Verification items for this drawing (mm, ordinates from the low corner). Give positions to 0.01 mm unless a question says otherwise; leave off trailing zeros. Order: outer loops, then holes, each group sorted by start corner. A loop starts at its lowest first (then second) coordinate and runs counter-clockwise, first axis right, second up.
(1) Scan lines: L1, parallel to Z at x = 252, y = 0.35; L2, parallel to X at y = 0.55, z = 34.5. Record each from-to range of solid material in increasing order.
(2) Sectioned sample at A-A on y = 1.2. Record the cut outline in (x, z).
(3) Gauge pin test, flat ends, axial feed: pin 1 (1 mm diameter, centred on x = 91, z = 36.5, fed in from -Y); pin 2 (1.5 mm diameter, centred on y = 2, z = 88.5, fed in from +X); pin 3 (1.5 mm diameter, centred on y = 2, z = 88.5, fed in from -X). Record the tip position at first contact, or that the pin passes through.
(4) Sectioned sample at B-B on x = 169.5. Record the cut outline in (y, z), plus the area to 3 significant figures.
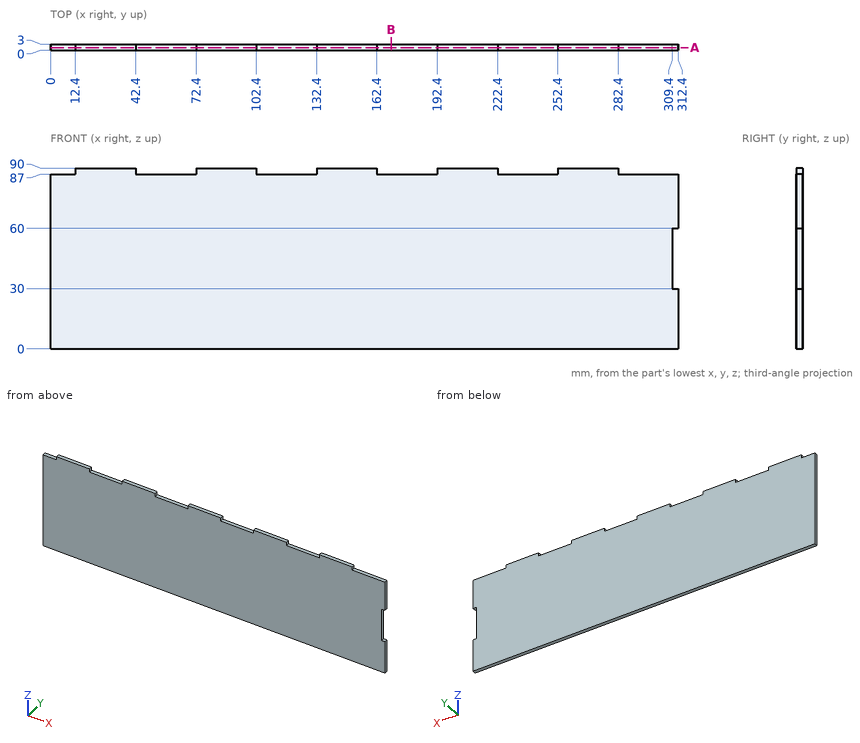
Ans:
1. L1: z = 0 to 87
1. L2: x = 0 to 309.4
2. outline: (0, 0) - (312.4, 0) - (312.4, 30) - (309.4, 30) - (309.4, 60) - (312.4, 60) - (312.4, 87) - (282.4, 87) - (282.4, 90) - (252.4, 90) - (252.4, 87) - (222.4, 87) - (222.4, 90) - (192.4, 90) - (192.4, 87) - (162.4, 87) - (162.4, 90) - (132.4, 90) - (132.4, 87) - (102.4, 87) - (102.4, 90) - (72.4, 90) - (72.4, 87) - (42.4, 87) - (42.4, 90) - (12.4, 90) - (12.4, 87) - (0, 87) - close
3. pin 1: stops at y = 0
3. pin 2: stops at x = 282.4
3. pin 3: stops at x = 12.4
4. outline: (0, 0) - (3, 0) - (3, 87) - (0, 87) - close
4. area: 261 mm2
